```python
from build123d import *

# Parameters (mm, degrees)
SKETCH1_W                   = 25.4
SKETCH1_H                   = 80
BOSS_EXTRUDE1_DEPTH         = 25.4
F_1_4_0_25_DIAMETER_HOLE1_D = 6.35
SKETCH4_W                   = 20.4
SKETCH4_H                   = 2
CUT_EXTRUDE1_DEPTH          = 88.694469609
M6_CLEARANCE_HOLE1_REACH    = 89.694
M6_CLEARANCE_HOLE1_BORE_R   = 3.3
M6X1_0_TAPPED_HOLE1_D       = 5
M6X1_0_TAPPED_HOLE1_DEPTH   = 17
M6X1_0_TAPPED_HOLE1_TIP     = 1.502151548
M8X1_25_TAPPED_HOLE1_D      = 6.8
M6X1_0_TAPPED_HOLE2_D       = 5


with BuildPart() as part:
    # Sketch1 → Boss-Extrude1 (new body)
    with BuildSketch(Plane(origin=(0, 0, 0), x_dir=(1, 0, 0), z_dir=(0, 1, 0))):
        with Locations((12.7, 40)):
            Rectangle(SKETCH1_W, SKETCH1_H)
    extrude(amount=BOSS_EXTRUDE1_DEPTH)

    # 1/4 (0.25) Diameter Hole1 (through all)
    with Locations(Plane(origin=(0, 25.4, 0), x_dir=(1, 0, 0), z_dir=(0, 1, 0))):
        with Locations((20.4, 10)):
            Hole(F_1_4_0_25_DIAMETER_HOLE1_D / 2)

    # Sketch4 → Cut-Extrude1 (cut, through all)
    with BuildSketch(Plane(origin=(0, 25.4, 0), x_dir=(1, 0, 0), z_dir=(0, 1, 0))):
        with Locations((10.2, 10)):
            Rectangle(SKETCH4_W, SKETCH4_H)
    extrude(amount=-CUT_EXTRUDE1_DEPTH, mode=Mode.SUBTRACT)

    # M6 Clearance Hole1 bore → M6 Clearance Hole1 (cut, up to next)
    with BuildSketch(Plane.XY, mode=Mode.PRIVATE) as m6_clearance_hole1_sk1:
        with Locations((5, 12.7)):
            Circle(M6_CLEARANCE_HOLE1_BORE_R)
    m6_clearance_hole1_tool1 = extrude(m6_clearance_hole1_sk1.sketch, amount=-M6_CLEARANCE_HOLE1_REACH, mode=Mode.PRIVATE) & part.part
    add(m6_clearance_hole1_tool1.solids().sort_by_distance((5, 12.7, 0))[0], mode=Mode.SUBTRACT)

    # M6x1.0 Tapped Hole1
    with Locations(Plane.XY.offset(-11)):
        with Locations((5, 12.7)):
            Hole(M6X1_0_TAPPED_HOLE1_D / 2, depth=M6X1_0_TAPPED_HOLE1_DEPTH)
            with Locations((0, 0, -(M6X1_0_TAPPED_HOLE1_DEPTH + M6X1_0_TAPPED_HOLE1_TIP / 2))):  # 118° drill point
                Cone(0, M6X1_0_TAPPED_HOLE1_D / 2, M6X1_0_TAPPED_HOLE1_TIP, mode=Mode.SUBTRACT)

    # M8x1.25 Tapped Hole1 (through all)
    with Locations(Plane(origin=(0, 25.4, 0), x_dir=(1, 0, 0), z_dir=(0, 1, 0))):
        with Locations((12.7, 70)):
            Hole(M8X1_25_TAPPED_HOLE1_D / 2)

    # M6x1.0 Tapped Hole2 (through all)
    with Locations(Plane(origin=(0, 0, 0), x_dir=(-1, 0, 0), z_dir=(0, -1, 0))):
        with Locations((-12.7, 26), (-12.7, 46)):
            Hole(M6X1_0_TAPPED_HOLE2_D / 2)


solid = part.part
```
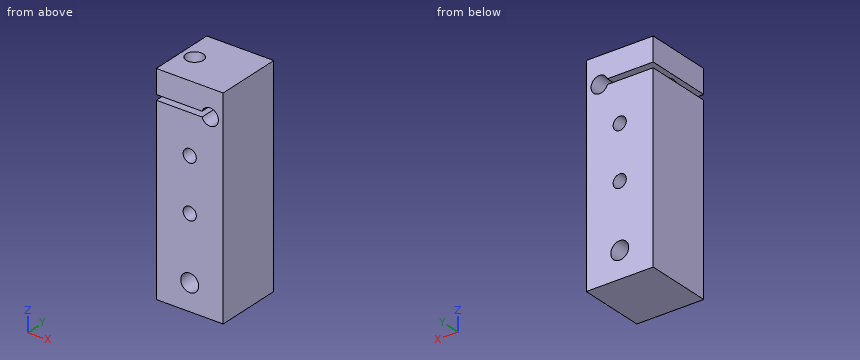
Input: part model. Units: mm. Frame: model coordinates. Coordinates: 2 decimals unless noted, no trailing zeros. Write each loop counter-clockwise with the first axis right and the second up, starting at its lowest first coordinate (ties: lowest second). Pieces come first, ordered by that corner, then holes. Notation, with made-up numbers: (-8, 50) -> (3, 50) arc R33 ccw to (3, 84) -> close; hole circle Ø1 at (78.25, 27.5). An arc over 180 degrees is marked (long way). Answer as a JSON object with one key per item and string values.
1. Material intervals for line 1 (Z direction, x = 12.7, y = 18.5); line 2 (Y direction, x = 5, z = -5); line 3 (Z direction, x = 1.5, y = 16), sorted ascending. Write a range as from..to.
Result set:
{"line 1": "z = -80..-73.4, -66.6..-48.5, -43.5..-28.5, -23.5..-11, -9..0", "line 2": "y = 0..9.4, 16..25.4", "line 3": "z = -80..-11, -9..0"}
2. Section C-C on x = 12.7. Return the cut outline in (y, z).
Result set:
{"outline": "(0, -80) -> (25.4, -80) -> (25.4, -73.4) -> (0, -73.4) -> close; (0, -66.6) -> (25.4, -66.6) -> (25.4, -48.5) -> (0, -48.5) -> close; (0, -43.5) -> (25.4, -43.5) -> (25.4, -28.5) -> (0, -28.5) -> close; (0, -23.5) -> (25.4, -23.5) -> (25.4, -11) -> (0, -11) -> close; (0, -9) -> (25.4, -9) -> (25.4, 0) -> (0, 0) -> close"}
3. Section D-D on z = -46. Return the cut outline in (x, y).
Result set:
{"outline": "(0, 0) -> (10.2, 0) -> (10.2, 25.4) -> (0, 25.4) -> close; (15.2, 0) -> (25.4, 0) -> (25.4, 25.4) -> (15.2, 25.4) -> close"}
4. First-contact query: P1, Ø11, axis at x = 12.7, z = -70, coming from the +Y side; P2, Ø4.5, axis at x = 5, y = 12.7, coming from the +Z side. Flat tips, straight axial feed; report the tip coordinate or a pass-through.
Result set:
{"P1": "stops at y = 25.4", "P2": "stops at z = -28.15"}
5. Section A-A on z = -26. Return the cut outline in (x, y), then the cut area to 3 significant figures.
Result set:
{"outline": "(0, 0) -> (10.2, 0) -> (10.2, 25.4) -> (0, 25.4) -> close; (15.2, 0) -> (25.4, 0) -> (25.4, 25.4) -> (15.2, 25.4) -> close; hole circle Ø5 at (5, 12.7)", "area": "499 mm2"}
6. Section B-B on x = 20.4. Return the cut outline in (y, z) (3 decimals), then the cut area to 3 significant figures.
Result set:
{"outline": "(0, -80) -> (25.4, -80) -> (25.4, -13.175) -> (0, -13.175) -> close; (0, -6.825) -> (25.4, -6.825) -> (25.4, 0) -> (0, 0) -> close", "area": "1,870 mm2"}
